Source: three-view drawing plus pictorial views. Frame: mm from the lowest corner of the part. Coordinates: 2 decimals unless noted, no trailing zeros. Order: outer loops, then holes, each group sorted by start corner. A loop starts at its lowest first (then second) coordinate and runs counter-clockwise, first axis right, second up. Notation, with made-up numbers: M 6.5,81 L 15.5,81 A20 ccw 15.5,110 Z; hole C 71.5,51.25 d10. An arc over 180 degrees is marked long. One line per question, with ' | ' between items.
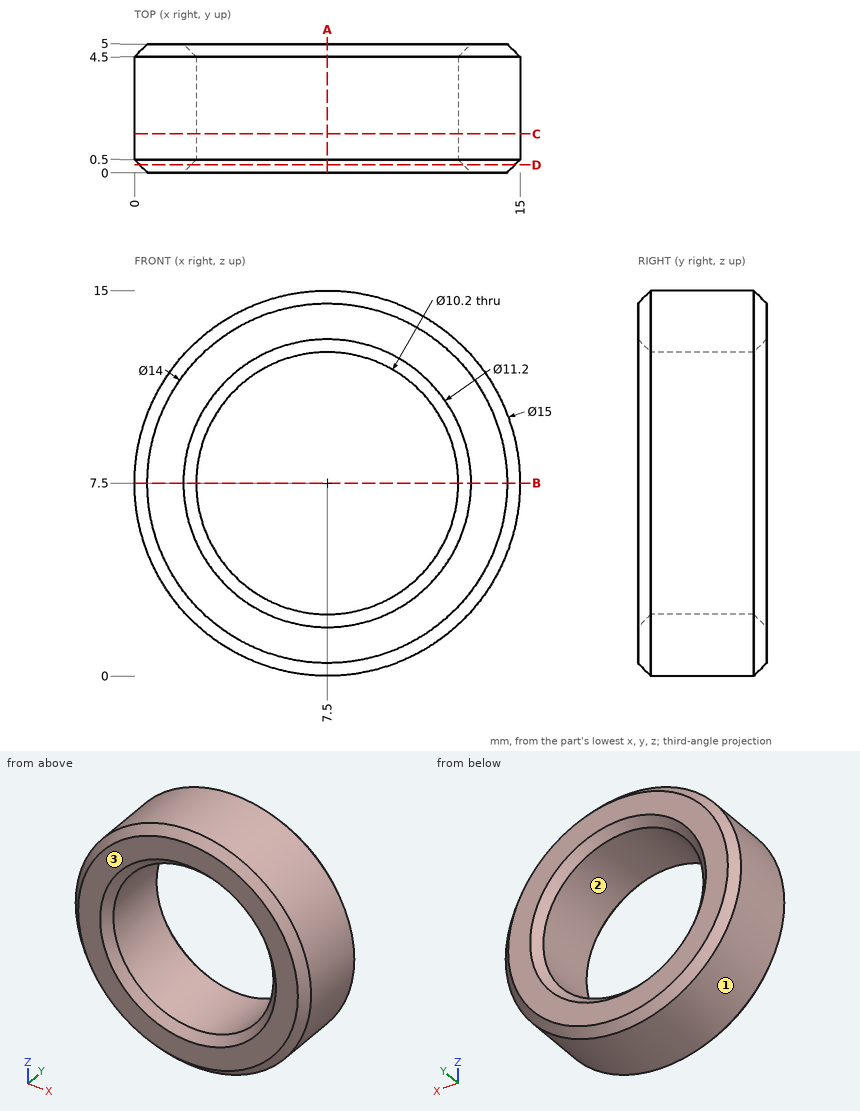
1. Section B-B, the plane z = 7.5. Output: boundary loops of the cut face in (x, y), and give its area (3 significant figures).
Response values:
outline: M 0,0.5 L 0.5,0 L 1.9,0 L 2.4,0.5 L 2.4,4.5 L 1.9,5 L 0.5,5 L 0,4.5 Z; M 12.6,0.5 L 13.1,0 L 14.5,0 L 15,0.5 L 15,4.5 L 14.5,5 L 13.1,5 L 12.6,4.5 Z | area: 23.0 mm^2
2. Section C-C, the plane y = 1.5. Output: boundary loops of the cut face in (x, z).
Response values:
outline: C 7.5,7.5 d15; hole C 7.5,7.5 d10.2
3. Section A-A, the plane x = 7.5. Output: boundary loops of the cut face in (y, z), and give its area (3 significant figures).
Response values:
outline: M 0,0.5 L 0.5,0 L 4.5,0 L 5,0.5 L 5,1.9 L 4.5,2.4 L 0.5,2.4 L 0,1.9 Z; M 0,13.1 L 0.5,12.6 L 4.5,12.6 L 5,13.1 L 5,14.5 L 4.5,15 L 0.5,15 L 0,14.5 Z | area: 23.0 mm^2
4. Section D-D, the plane y = 0.3. Output: boundary loops of the cut face in (x, z), and give its area (3 significant figures).
Response values:
outline: C 7.5,7.5 d14.6; hole C 7.5,7.5 d10.6 | area: 79.2 mm^2
5. Pin query (flat end, axial travel): P1, Ø2, axis at y = 3, z = 3.5, coming from the -X side; P2, Ø1, axis at x = 12.5, y = 1, coming from the +Z side; P3, Ø2, axis at y = 3, z = 11, coming from the +X side. Return the tip coordinate at first contact, or that it passes through.
Response values:
P1: stops at x = 0.63 | P2: stops at z = 13.5 | P3: stops at x = 14.57
6. Draft query along Z for the marked faces 1, 2 and 3. Return one class per face: pulls with the +Z half, pulls with the -Z half, needs draft (parallel to the pull), parting line crosses it, or undercut.
Response values:
face 1: parting line crosses it | face 2: undercut | face 3: needs draft
7. Material intervals for line 1 (Z direction, x = 7.5, y = 3.2); line 2 (Z direction, x = 6, y = 0.3); line 3 (X direction, y = 0.9, z = 11.5), sorted ascending. Write a range as [from, to].
Response values:
line 1: z = [0, 2.4], [12.6, 15] | line 2: z = [0.36, 2.42], [12.58, 14.64] | line 3: x = [1.16, 4.34], [10.66, 13.84]
